Autodesk Inventor part; units mm, degrees
ref_plane "YZ Plane" through (0, 0, 0) normal (1, 0, 0) x (0, 1, 0)
ref_plane "XZ Plane" through (0, 0, 0) normal (0, 1, 0) x (-1, 0, 0)
ref_plane "XY Plane" through (0, 0, 0) normal (0, 0, 1) x (1, 0, 0)
sketch "Sketch1" plane through (0, 0, 0) normal (0, 0, 1) x (1, 0, 0)
  line L0 (0, 0) -> (76.2, 0)
  line L1 (76.2, 0) -> (76.2, 139.7)
  line L2 (76.2, 139.7) -> (0, 139.7)
  line L3 (0, 139.7) -> (0, 0)
  line L4 (15.6073, 25.4999) -> (15.6073, 120.9664)
  arc A0 (34.9423, 120.9664) -> (15.6073, 120.9664) centre (25.2748, 120.9664) ccw
  line L5 (34.9423, 120.9664) -> (34.9423, 25.4999)
  arc A1 (15.6073, 25.4999) -> (34.9423, 25.4999) centre (25.2748, 25.4999) ccw
  line L6 (2.202, 137.498) -> (73.998, 137.498)
  line L7 (73.998, 137.498) -> (73.998, 2.202)
  line L8 (73.998, 2.202) -> (2.202, 2.202)
  line L9 (2.202, 2.202) -> (2.202, 137.498)
  dimension "d0" = 76.2
  dimension "d1" = 139.7
extrude "Extrusion1" add sketch "Sketch1" against normal blind 4.7625 contours L3 L2 L1 L0 | L6 L7 L8 L9
extrude "Extrusion2" add sketch "Sketch1" along normal blind 3.81 contours L6 L7 L8 L9
properties part number "Shifter surround"
Work out the finished part from the listing and answer in its coordinate system (mm). A direction names the side the tool comes from. Round coordinates to 2 decimals unless told otherwise and drop trailing zeros. Order: outer loops, then holes, each group sorted by start corner. A loop starts at its lowest first (then second) coordinate and runs counter-clockwise, first axis right, second up. Notation, with made-up numbers: M 55,53 L 106,53 A14 ccw 106,58 Z; hole C -24,-1.5 d3. An arc over 180 degrees is marked long. Put each result on its own line as item: value. Start each with the question number.
Q1. A tool of negligible diameter and unlimited length cuts with its end or side. For faces 5 (the flat face through (39, 2.202, 2)), 6 (the flat face through (73.998, 71, 2)), 7 (the flat face through (34.942, 74, -1)), 8 (the flat face through (2.202, 69, 2)), from which of +Z, -Z, +X, -X, +Y, -Y can it reach the whole face along a straight path? Write none if from no direction.
Q2. Section C-C, the plane x = 27.5 is taken. Write down the section's boundary in (y, z), and give its area (3 significant figures).
Q3. Section D-D, the plane y = 14 is taken. Write down the section's boundary in (x, z), and give its area (3 significant figures).
Q4. Section B-B, the plane y = 51.5 is taken. Write down the section's boundary in (x, z).
Q5. Section A-A, the plane z = 1.5 is taken. Write down the section's boundary in (x, y) (1 decimal), and give its area (3 significant figures).
Q6. Straight lines are drawn through the part: L1, parallel to X at y = 92, z = 3.5; L2, parallel to X at y = 95.5, z = -2; L3, parallel to Y at x = 59.5, z = 1.5. For each, find the intervals that lie inside material, in ascending order. Write a range as [from, to].
Q7. For a pull along X with two mould halves and no side action, classify faces 1 (the cylindrical face through (25.06, 130.63, -0.54)), 2 (the flat face through (38, 71, 3.81)), 3 (the flat face through (0, 71, -2)), 4 (the flat face through (15.607, 73, -1)) as pulls with the +X half, pulls with the -X half, needs draft (parallel to the pull), parting line crosses it, or undercut.
Q8. Flat-ended cylindrical pins translate along their axes: pin 1 (1.9 mm diameter, centred on x = 36, z = 1.5, fed in from +Y); pin 2 (1.9 mm diameter, centred on y = 91, z = 1.5, fed in from -X); pin 3 (2 mm diameter, centred on x = 45.5, z = 1.5, fed in from -Y). Find the tip coordinate at first contact, or state that the pin passes through.
Findings below:
1. face 5: +Z, +X, -X, -Y
1. face 6: +Z, +X, +Y, -Y
1. face 7: +Z, -Z
1. face 8: +Z, -X, +Y, -Y
2. outline: M 0,-4.76 L 16.09,-4.76 L 16.09,3.81 L 2.2,3.81 L 2.2,0 L 0,0 Z; M 130.37,-4.76 L 139.7,-4.76 L 139.7,0 L 137.5,0 L 137.5,3.81 L 130.37,3.81 Z
2. area: 201 mm^2
3. outline: M 0,-4.76 L 76.2,-4.76 L 76.2,0 L 74,0 L 74,3.81 L 2.2,3.81 L 2.2,0 L 0,0 Z
3. area: 636 mm^2
4. outline: M 0,-4.76 L 15.61,-4.76 L 15.61,3.81 L 2.2,3.81 L 2.2,0 L 0,0 Z; M 34.94,-4.76 L 76.2,-4.76 L 76.2,0 L 74,0 L 74,3.81 L 34.94,3.81 Z
5. outline: M 2.2,2.2 L 74,2.2 L 74,137.5 L 2.2,137.5 Z; hole M 15.6,25.5 A9.7 ccw 34.9,25.5 L 34.9,121 A9.7 ccw 15.6,121 Z
5. area: 7,570 mm^2
6. L1: x = [2.2, 15.61], [34.94, 74]
6. L2: x = [0, 15.61], [34.94, 76.2]
6. L3: y = [2.2, 137.5]
7. face 1: undercut
7. face 2: needs draft
7. face 3: pulls with the -X half
7. face 4: undercut
8. pin 1: stops at y = 137.5
8. pin 2: stops at x = 2.2
8. pin 3: stops at y = 2.2
